Can you work these out from the model? Positions are in its coordinate system, mm. Round coordinates to 2 decimals unless told otherwise and drop trailing zeros. Loops run counter-clockwise (first coordinate to the right, second up) from the corner with the lowest first, then second, coordinate; pieces in that order, holes last. Notation, with made-up numbers: (39, -25) - (47, -25) arc R21 cw to (47, 14) - close; hole circle Ø9 at (71, -3). An arc over 180 degrees is marked (long way). Answer as CSV lines item,"result".
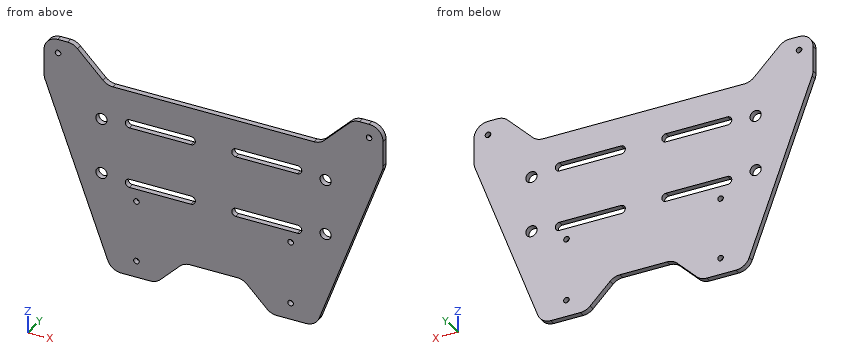
```python
from build123d import *

# Parameters (mm, degrees)
SKETCH1_W                = 130
SKETCH1_H                = 90
BOSS_EXTRUDE2_DEPTH      = 2
SKETCH2_R                = 2
CUT_EXTRUDE1_DEPTH       = 10
CUT_EXTRUDE3_DEPTH       = 10
SKETCH5_R                = 1
CUT_EXTRUDE4_DEPTH       = 10
SKETCH7_W                = 130
SKETCH7_H                = 10
CUT_EXTRUDE5_DEPTH       = 10
CUT_EXTRUDE10_DEPTH      = 149.761308663
CUT_EXTRUDE10_DEPTH_BACK = 149.761308663
CUT_EXTRUDE14_DEPTH      = 149.761308663
CUT_EXTRUDE14_DEPTH_BACK = 13
SKETCH12_R               = 1
FILLET2_R                = 5


with BuildPart() as part:
    # Sketch1 → Boss-Extrude2 (new body)
    with BuildSketch(Plane(origin=(0, 0, 0), x_dir=(1, 0, 0), z_dir=(0, 1, 0))):
        with Locations((56.787418592, 40.403463793)):
            Rectangle(SKETCH1_W, SKETCH1_H)
    extrude(amount=BOSS_EXTRUDE2_DEPTH)

    # Sketch2 → Cut-Extrude1 (cut)
    with BuildSketch(Plane(origin=(0, 2, 0), x_dir=(1, 0, 0), z_dir=(0, 1, 0))):
        with Locations(Location((16.787418592, 50.403463793, 0), (0, 0, 270))):
            Circle(SKETCH2_R)
        with Locations(Location((16.787418592, 30.403463793, 0), (0, 0, 270))):
            Circle(SKETCH2_R)
        with Locations(Location((96.787418592, 50.403463793, 0), (0, 0, 270))):
            Circle(SKETCH2_R)
        with Locations(Location((96.787418592, 30.403463793, 0), (0, 0, 270))):
            Circle(SKETCH2_R)
    extrude(amount=-CUT_EXTRUDE1_DEPTH, mode=Mode.SUBTRACT)

    # Sketch4 → Cut-Extrude3 (cut)
    with BuildSketch(Plane(origin=(0, 2, 0), x_dir=(1, 0, 0), z_dir=(0, 1, 0))):
        with BuildLine():
            Line((26.787418592, 52.903463793), (48.787418592, 52.903463793))
            ThreePointArc((48.787418592, 52.903463793), (50.287418592, 51.403463793), (48.787418592, 49.903463793))
            Line((48.787418592, 49.903463793), (26.787418592, 49.903463793))
            ThreePointArc((26.787418592, 49.903463793), (25.287418592, 51.403463793), (26.787418592, 52.903463793))
        make_face()
        with BuildLine():
            Line((26.787418592, 30.903463793), (48.787418592, 30.903463793))
            ThreePointArc((48.787418592, 30.903463793), (50.287418592, 29.403463793), (48.787418592, 27.903463793))
            Line((48.787418592, 27.903463793), (26.787418592, 27.903463793))
            ThreePointArc((26.787418592, 27.903463793), (25.287418592, 29.403463793), (26.787418592, 30.903463793))
        make_face()
        with BuildLine():
            Line((64.787418592, 52.903463793), (86.787418592, 52.903463793))
            ThreePointArc((86.787418592, 52.903463793), (88.287418592, 51.403463793), (86.787418592, 49.903463793))
            Line((86.787418592, 49.903463793), (64.787418592, 49.903463793))
            ThreePointArc((64.787418592, 49.903463793), (63.287418592, 51.403463793), (64.787418592, 52.903463793))
        make_face()
        with BuildLine():
            Line((64.787418592, 30.903463793), (86.787418592, 30.903463793))
            ThreePointArc((86.787418592, 30.903463793), (88.287418592, 29.403463793), (86.787418592, 27.903463793))
            Line((86.787418592, 27.903463793), (64.787418592, 27.903463793))
            ThreePointArc((64.787418592, 27.903463793), (63.287418592, 29.403463793), (64.787418592, 30.903463793))
        make_face()
    extrude(amount=-CUT_EXTRUDE3_DEPTH, mode=Mode.SUBTRACT)

    # Sketch5 → Cut-Extrude4 (cut)
    with BuildSketch(Plane(origin=(0, 2, 0), x_dir=(1, 0, 0), z_dir=(0, 1, 0))):
        with Locations(Location((1.287418592, 10.403463793, 0), (0, 0, 270))):
            Circle(SKETCH5_R)
        with Locations(Location((112.287418592, 10.403463793, 0), (0, 0, 270))):
            Circle(SKETCH5_R)
        with Locations(Location((84.287418592, 56.920801797, 0), (0, 0, 270))):
            Circle(SKETCH5_R)
        with Locations(Location((116.787418592, 57.403463793, 0), (0, 0, 270))):
            Circle(SKETCH5_R)
        with Locations(Location((116.787418592, 79.403463793, 0), (0, 0, 270))):
            Circle(SKETCH5_R)
        with Locations(Location((84.287418592, 79.403463793, 0), (0, 0, 270))):
            Circle(SKETCH5_R)
        with Locations(Location((-3.212581408, 57.403463793, 0), (0, 0, 270))):
            Circle(SKETCH5_R)
        with Locations(Location((29.287418592, 57.403463793, 0), (0, 0, 270))):
            Circle(SKETCH5_R)
        with Locations(Location((29.287418592, 79.403463793, 0), (0, 0, 270))):
            Circle(SKETCH5_R)
        with Locations(Location((-3.212581408, 79.403463793, 0), (0, 0, 270))):
            Circle(SKETCH5_R)
    extrude(amount=-CUT_EXTRUDE4_DEPTH, mode=Mode.SUBTRACT)

    # Sketch7 → Cut-Extrude5 (cut)
    with BuildSketch(Plane(origin=(0, 2, 0), x_dir=(1, 0, 0), z_dir=(0, 1, 0))):
        with Locations((56.787418592, 0.403463793)):
            Rectangle(SKETCH7_W, SKETCH7_H)
    extrude(amount=-CUT_EXTRUDE5_DEPTH, mode=Mode.SUBTRACT)

    # Sketch9 → Cut-Extrude10 (cut, two sides: drawn at the far end of the back side and taken through both)
    with BuildSketch(Plane(origin=(0, 2, 0), x_dir=(1, 0, 0), z_dir=(0, 1, 0)).offset(-CUT_EXTRUDE10_DEPTH_BACK)):
        Polygon((-198.399776781, -199.78373158), (6.787418592, 5.403463793), (18.787418592, 17.403463793), (94.787418592, 17.403463793), (106.787418592, 5.403463793), (311.974613966, -199.78373158), (311.974613966, -780.140760625), (-198.399776781, -780.140760625), align=None)
    extrude(amount=CUT_EXTRUDE10_DEPTH + CUT_EXTRUDE10_DEPTH_BACK, mode=Mode.SUBTRACT)

    # Sketch12 → Cut-Extrude14 (cut, two sides: drawn at the far end of the back side and taken through both)
    # profile 1 of 3: a face of its own
    with BuildSketch(Plane(origin=(0, 2, 0), x_dir=(1, 0, 0), z_dir=(0, 1, 0)).offset(-CUT_EXTRUDE14_DEPTH_BACK)):
        Polygon((-8.212581408, 5.403463793), (-3.712581408, 5.403463793), (-3.712581408, 20.403463793), (20.287418592, 85.403463793), (-8.212581408, 85.403463793), align=None)
        with Locations((-3.212581408, 57.403463793)):
            Circle(SKETCH12_R, mode=Mode.SUBTRACT)
        with Locations((-3.212581408, 79.403463793)):
            Circle(SKETCH12_R, mode=Mode.SUBTRACT)
    # profile 2 of 3: a face of its own
    with BuildSketch(Plane(origin=(0, 2, 0), x_dir=(1, 0, 0), z_dir=(0, 1, 0)).offset(-CUT_EXTRUDE14_DEPTH_BACK)):
        Polygon((77.287418592, 85.403463793), (36.287418592, 85.403463793), (46.287418592, 75.403463793), (67.287418592, 75.403463793), align=None)
    # profile 3 of 3: a face of its own
    with BuildSketch(Plane(origin=(0, 2, 0), x_dir=(1, 0, 0), z_dir=(0, 1, 0)).offset(-CUT_EXTRUDE14_DEPTH_BACK)):
        Polygon((121.787418592, 85.403463793), (93.287418592, 85.403463793), (117.287418592, 20.403463793), (117.287418592, 5.403463793), (121.787418592, 5.403463793), align=None)
        with Locations((116.787418592, 57.403463793)):
            Circle(SKETCH12_R, mode=Mode.SUBTRACT)
        with Locations((116.787418592, 79.403463793)):
            Circle(SKETCH12_R, mode=Mode.SUBTRACT)
    extrude(amount=CUT_EXTRUDE14_DEPTH + CUT_EXTRUDE14_DEPTH_BACK, mode=Mode.SUBTRACT)

    # Fillet2
    fillet2_edges = [part.edges().sort_by_distance(p)[0] for p in [
        (-3.712581408, 1, -5.403463793),
        (-3.712581408, 1, -20.403463793),
        (18.787418592, 1, -17.403463793),
        (6.787418592, 1, -5.403463793),
        (94.787418592, 1, -17.403463793),
        (106.787418592, 1, -5.403463793),
        (117.287418592, 1, -5.403463793),
        (117.287418592, 1, -20.403463793),
        (93.287418592, 1, -85.403463793),
        (20.287418592, 1, -85.403463793),
        (36.287418592, 1, -85.403463793),
        (46.287418592, 1, -75.403463793),
        (67.287418592, 1, -75.403463793),
        (77.287418592, 1, -85.403463793),
    ]]
    fillet(fillet2_edges, radius=FILLET2_R)


solid = part.part
```
Q1. Imagine slicing it at B-B (z = -14). Write out the boundary of the cut face in (x, y).
Checks:
outline,"(-3.71, 0) - (15.38, 0) - (15.38, 2) - (-3.71, 2) - close; (98.19, 0) - (117.29, 0) - (117.29, 2) - (98.19, 2) - close"
Q2. If I drill on line 1 along X through (y, z) = (0.65, -30); line 2 along Z through (x, y) = (70, 1.05); line 3 along Z through (x, y) = (88, 0.65), over which ranges is the centre line in solid material (lowest first)? Write a range as [from, to].
Checks:
line 1,"[-0.17, 14.83], [18.75, 25.41], [50.16, 63.41], [88.16, 94.83], [98.75, 113.74]"
line 2,"[-78.12, -52.9], [-49.9, -30.9], [-27.9, -17.4]"
line 3,"[-85.4, -52.29], [-50.52, -30.29], [-28.52, -17.4]"
Q3. I'm going to push flat-ended pins straight in: pin 1 Ø1 at (x, y) = (40, 0.5) entering from +Z; pin 2 Ø1 at (x, y) = (74, 0.5) entering from -Z. Where does each tip first touch, or does it pass through?
Checks:
pin 1,"z = -17.4"
pin 2,"z = -82.62"
Q4. Imagine slicing it at C-C (y = 0.35). Count the separate pieces of the cut face and the enclosed holes in it, then the cut area to 3 significant figures.
Checks:
separate pieces,"1"
enclosed holes,"14"
area,"6,380 mm²"
Q5. Imagine slicing it at D-D (x = 103.5). Write out the boundary of the cut face in (y, z).
Checks:
outline,"(0, -57.74) - (2, -57.74) - (2, -8.69) - (0, -8.69) - close"
Q6. Imagine slicing it at A-A (x = 46.5). Write out the boundary of the cut face in (y, z), then the cut area to 3 significant figures.
Checks:
outline,"(0, -75.76) - (2, -75.76) - (2, -52.9) - (0, -52.9) - close; (0, -49.9) - (2, -49.9) - (2, -30.9) - (0, -30.9) - close; (0, -27.9) - (2, -27.9) - (2, -17.4) - (0, -17.4) - close"
area,"105 mm²"
